Part model, mm, in its own coordinate system. Face numbers are marked on the shaded views. Round coordinates to 2 decimals unless told otherwise and drop trailing zeros. Loops run counter-clockwise (first coordinate to the right, second up) from the corner with the lowest first, then second, coordinate; pieces in that order, holes last. Notation, with made-up numbers: (59, 66) -> (98, 66) arc R20 cw to (98, 78) -> close; hole circle Ø2 at (-33.75, -33). An arc over 180 degrees is marked (long way). Use a Markdown table: item, result. Add a question column.
Item 1: Probe line 1 (Y direction, x = 28, z = 4); line 2 (Y direction, x = -1, z = 6.25); line 3 (Z direction, x = -15.5, y = 9). List the from-to ranges inside material, lowest first. Write a range as [from, to].
Item 2: Flat gauge pins, fed straight in: pin 1 (1 mm diameter, centred on x = -1.5, z = 8, fed in from -Y); pin 2 (2.5 mm diameter, centred on x = 3, y = 17.5, fed in from +Z). Where does each tip first touch, or does it go through?
Item 3: Cut at D-D, the plane y = 5. List the corners of the cut face in (x, z), plus the area to 3 significant figures.
Item 4: Two-plate mould, pull along Y, no slides. Class the marked faces 1, 2 and 3: pulls with the +Y half, pulls with the -Y half, needs draft (parallel to the pull), parting line crosses it, or undercut.
Item 5: Cut at C-C, the plane z = 9.5. List the corners of the cut face in (x, y).
Item 6: Cut at A-A, the plane y = -16.8. List the corners of the cut face in (x, z).
Item 7: Cut at B-B, the plane x = 11. List the corners of the cut face in (y, z), plus the area to 3 significant figures.
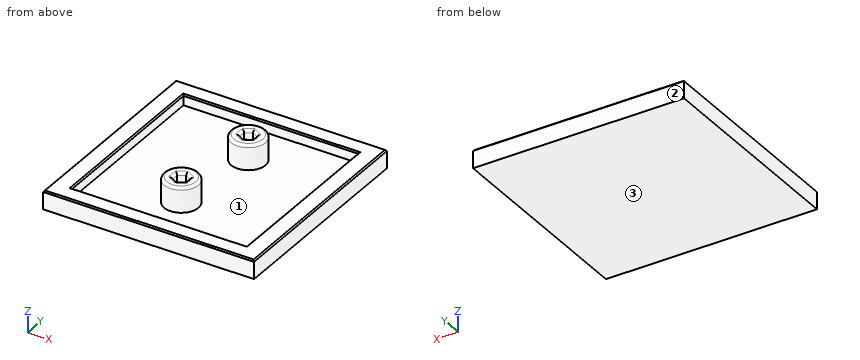
```python
from build123d import *

# Parameters (mm, degrees)
F0_W     = 80
F0_H     = 80
F0_R     = 6.5
F1_DEPTH = 3
F2_DEPTH = 12.5
F3_R     = 1
F4_W     = 80
F4_H     = 80
F4_W_2   = 66.2
F4_H_2   = 67.2
F5_DEPTH = 4
F6_SIZE  = 0.5


# Not quite as in the source:
# - a feature names something its author has since deleted; it is built from what else it names


with BuildPart() as f1:
    # F0 (on Top) → F1 (new body)
    with BuildSketch(Plane.XY):
        Rectangle(F0_W, F0_H)
        with Locations((-2.17, -16.8)):
            Circle(F0_R, mode=Mode.SUBTRACT)
        with Locations((2.17, 16.617)):
            Circle(F0_R, mode=Mode.SUBTRACT)
        with Locations((2.17, 16.617)):
            Circle(F0_R)
        Polygon((-0.3917684664, 18.0686688068), (2.1462978314, 19.5613909739), (4.7080662978, 18.1097221671), (4.7317684664, 15.1653311932), (2.1937021686, 13.6726090261), (-0.3680662978, 15.1242778329), align=None, mode=Mode.SUBTRACT)
        Polygon((4.7080662978, 18.1097221671), (2.1462978314, 19.5613909739), (-0.3917684664, 18.0686688068), (-0.3680662978, 15.1242778329), (2.1937021686, 13.6726090261), (4.7317684664, 15.1653311932), align=None)
        with Locations((-2.17, -16.8)):
            Circle(F0_R)
        Polygon((-2.17, -13.8555136271), (0.38, -15.3277568136), (0.38, -18.2722431864), (-2.17, -19.7444863729), (-4.72, -18.2722431864), (-4.72, -15.3277568136), align=None, mode=Mode.SUBTRACT)
        Polygon((0.38, -18.2722431864), (0.38, -15.3277568136), (-2.17, -13.8555136271), (-4.72, -15.3277568136), (-4.72, -18.2722431864), (-2.17, -19.7444863729), align=None)
    extrude(amount=F1_DEPTH)

    # F0 (on Top) → F2 (join)
    with BuildSketch(Plane.XY):
        with Locations((2.17, 16.617)):
            Circle(F0_R)
        Polygon((-0.3917684664, 18.0686688068), (2.1462978314, 19.5613909739), (4.7080662978, 18.1097221671), (4.7317684664, 15.1653311932), (2.1937021686, 13.6726090261), (-0.3680662978, 15.1242778329), align=None, mode=Mode.SUBTRACT)
        with Locations((-2.17, -16.8)):
            Circle(F0_R)
        Polygon((-2.17, -13.8555136271), (0.38, -15.3277568136), (0.38, -18.2722431864), (-2.17, -19.7444863729), (-4.72, -18.2722431864), (-4.72, -15.3277568136), align=None, mode=Mode.SUBTRACT)
    extrude(amount=F2_DEPTH)

    # F3
    f3_edges = [f1.edges().sort_by_distance(p)[0] for p in [
        (-4.33, 16.617, 12.5),
        (0.877265, 18.81503, 12.5),
        (3.427182, 18.835557, 12.5),
        (4.719917, 16.637527, 12.5),
        (3.462735, 14.41897, 12.5),
        (0.912818, 14.398443, 12.5),
        (-0.379917, 16.596473, 12.5),
        (-8.67, -16.8, 12.5),
        (-0.895, -14.591635, 12.5),
        (0.38, -16.8, 12.5),
        (-0.895, -19.008365, 12.5),
        (-3.445, -19.008365, 12.5),
        (-4.72, -16.8, 12.5),
        (-3.445, -14.591635, 12.5),
    ]]
    fillet(f3_edges, radius=F3_R)

    # F4 (on face) → F5 (join)
    with BuildSketch(Plane.XY.offset(3)):
        Rectangle(F4_W, F4_H)
        Rectangle(F4_W_2, F4_H_2, mode=Mode.SUBTRACT)
    extrude(amount=F5_DEPTH)

    # F6
    f6_edges = [f1.edges().sort_by_distance(p)[0] for p in [
        (0, -40, 7),
        (40, 0, 7),
        (0, 40, 7),
        (-40, 0, 7),
        (0, 33.6, 7),
        (33.1, 0, 7),
        (0, -33.6, 7),
        (-33.1, 0, 7),
    ]]
    chamfer(f6_edges, length=F6_SIZE)


solid = f1.part
```
A:
| question | item | result |
|---|---|---|
| 1 | line 1 | y = [-40, -33.6], [33.6, 40] |
| 1 | line 2 | y = [-40, -33.6], [-23.19, -19.07], [-14.53, -10.41], [10.94, 22.29], [33.6, 40] |
| 1 | line 3 | z = [0, 3] |
| 2 | pin 1 | stops at y = -23.3 |
| 2 | pin 2 | stops at z = 3 |
| 3 | outline | (-40, 0) -> (40, 0) -> (40, 6.5) -> (39.5, 7) -> (33.6, 7) -> (33.1, 6.5) -> (33.1, 3) -> (-33.1, 3) -> (-33.1, 6.5) -> (-33.6, 7) -> (-39.5, 7) -> (-40, 6.5) -> close |
| 3 | area | 295 mm^2 |
| 4 | face 1 | undercut |
| 4 | face 2 | pulls with the +Y half |
| 4 | face 3 | needs draft |
| 5 | outline | circle Ø13 at (-2.17, -16.8); circle Ø13 at (2.17, 16.62); hole (-4.72, -18.27) -> (-2.17, -19.74) -> (0.38, -18.27) -> (0.38, -15.33) -> (-2.17, -13.86) -> (-4.72, -15.33) -> close; hole (-0.39, 18.07) -> (-0.37, 15.12) -> (2.19, 13.67) -> (4.73, 15.17) -> (4.71, 18.11) -> (2.15, 19.56) -> close |
| 6 | outline | (-40, 0) -> (40, 0) -> (40, 6.5) -> (39.5, 7) -> (33.6, 7) -> (33.1, 6.5) -> (33.1, 3) -> (4.33, 3) -> (4.33, 11.5) arc R1 ccw to (3.33, 12.5) -> (1.38, 12.5) arc R1 ccw to (0.38, 11.5) -> (0.38, 3) -> (-4.72, 3) -> (-4.72, 11.5) arc R1 ccw to (-5.72, 12.5) -> (-7.67, 12.5) arc R1 ccw to (-8.67, 11.5) -> (-8.67, 3) -> (-33.1, 3) -> (-33.1, 6.5) -> (-33.6, 7) -> (-39.5, 7) -> (-40, 6.5) -> close |
| 7 | outline | (-40, 0) -> (40, 0) -> (40, 6.5) -> (39.5, 7) -> (34.1, 7) -> (33.6, 6.5) -> (33.6, 3) -> (-33.6, 3) -> (-33.6, 6.5) -> (-34.1, 7) -> (-39.5, 7) -> (-40, 6.5) -> close |
| 7 | area | 291 mm^2 |
